```python
from build123d import *

# Parameters (mm, degrees)
SKETCH1_R             = 3.5
BOSS_EXTRUDE1_DEPTH   = 6.35
SKETCH2_R             = 3.25
CUT_EXTRUDE1_DEPTH    = 7.35
LPATTERN1_COUNT       = 5
LPATTERN1_PITCH       = 20
FILLET1_R             = 10
SKETCH3_R             = 3.25
SKETCH3_R_2           = 1
CUT_EXTRUDE2_DEPTH    = 7.35
CHAMFER1_SIZE         = 4
CHAMFER1_SIZE2        = 3.477146951
CHAMFER1_PART_2_SIZE  = 4
CHAMFER1_PART_2_SIZE2 = 3.477146951
CHAMFER1_PART_3_SIZE  = 4
CHAMFER1_PART_3_SIZE2 = 3.477146951
CHAMFER1_PART_4_SIZE  = 4
CHAMFER1_PART_4_SIZE2 = 3.477146951


with BuildPart() as part:
    # Sketch1 → Boss-Extrude1 (new body)
    with BuildSketch(Plane.XY):
        with BuildLine():
            Line((-40, 47.5), (-8.864317001, 107.128594183))
            ThreePointArc((-8.864317001, 107.128594183), (0, 112.5), (8.864317001, 107.128594183))
            Line((8.864317001, 107.128594183), (40, 47.5))
            Line((40, 47.5), (40, -47.5))
            Line((40, -47.5), (-40, -47.5))
            Line((-40, -47.5), (-40, 47.5))
        make_face()
        with Locations((-15, 47.5)):
            Circle(SKETCH1_R, mode=Mode.SUBTRACT)
        with Locations((15, 47.5)):
            Circle(SKETCH1_R, mode=Mode.SUBTRACT)
        with Locations((-15, 27.5)):
            Circle(SKETCH1_R, mode=Mode.SUBTRACT)
        with Locations((15, 27.5)):
            Circle(SKETCH1_R, mode=Mode.SUBTRACT)
    extrude(amount=BOSS_EXTRUDE1_DEPTH)

    # Sketch2 → Cut-Extrude1 (cut, through all)
    with BuildSketch(Plane.XY.offset(6.35)):
        with Locations((30, -37.5)):
            Circle(SKETCH2_R)
        with Locations((-30, -37.5)):
            Circle(SKETCH2_R)
    cut_extrude1 = extrude(amount=-CUT_EXTRUDE1_DEPTH, mode=Mode.SUBTRACT)

    # LPattern1: Cut-Extrude1 ×5
    with Locations(*[(0, i * LPATTERN1_PITCH, 0) for i in range(1, LPATTERN1_COUNT)]):
        add(cut_extrude1, mode=Mode.SUBTRACT)

    # Fillet1
    fillet1_edges = [part.edges().sort_by_distance(p)[0] for p in [
        (40, 47.5, 3.175),
        (40, -47.5, 3.175),
        (-40, -47.5, 3.175),
        (-40, 47.5, 3.175),
    ]]
    fillet(fillet1_edges, radius=FILLET1_R)

    # Sketch3 → Cut-Extrude2 (cut, through all)
    with BuildSketch(Plane.XY.offset(6.35)):
        with Locations((-20, 62.5)):
            Circle(SKETCH3_R)
        with Locations((20, 62.5)):
            Circle(SKETCH3_R)
        with Locations((0, 102.5)):
            Circle(SKETCH3_R_2)
    extrude(amount=-CUT_EXTRUDE2_DEPTH, mode=Mode.SUBTRACT)

    # Chamfer1
    chamfer1_edges = [part.edges().sort_by_distance(p)[0] for p in [
        (-18.5, 47.5, 0),
    ]]
    chamfer1_side = [part.faces().sort_by_distance(p)[0] for p in [
        (-18.5, 47.5, 3.175),
    ]]
    chamfer(chamfer1_edges, length=CHAMFER1_SIZE, length2=CHAMFER1_SIZE2, reference=chamfer1_side[0])

    # Chamfer1 part 2
    chamfer1_part_2_edges = [part.edges().sort_by_distance(p)[0] for p in [
        (11.5, 47.5, 0),
    ]]
    chamfer1_part_2_side = [part.faces().sort_by_distance(p)[0] for p in [
        (11.5, 47.5, 3.175),
    ]]
    chamfer(chamfer1_part_2_edges, length=CHAMFER1_PART_2_SIZE, length2=CHAMFER1_PART_2_SIZE2, reference=chamfer1_part_2_side[0])

    # Chamfer1 part 3
    chamfer1_part_3_edges = [part.edges().sort_by_distance(p)[0] for p in [
        (-18.5, 27.5, 0),
    ]]
    chamfer1_part_3_side = [part.faces().sort_by_distance(p)[0] for p in [
        (-18.5, 27.5, 3.175),
    ]]
    chamfer(chamfer1_part_3_edges, length=CHAMFER1_PART_3_SIZE, length2=CHAMFER1_PART_3_SIZE2, reference=chamfer1_part_3_side[0])

    # Chamfer1 part 4
    chamfer1_part_4_edges = [part.edges().sort_by_distance(p)[0] for p in [
        (11.5, 27.5, 0),
    ]]
    chamfer1_part_4_side = [part.faces().sort_by_distance(p)[0] for p in [
        (11.5, 27.5, 3.175),
    ]]
    chamfer(chamfer1_part_4_edges, length=CHAMFER1_PART_4_SIZE, length2=CHAMFER1_PART_4_SIZE2, reference=chamfer1_part_4_side[0])


solid = part.part
```
Part model, mm, in its own coordinate system. Round coordinates to 2 decimals unless told otherwise and drop trailing zeros. Write each loop counter-clockwise with the first axis right and the second up, starting at its lowest first coordinate (ties: lowest second). Pieces come first, ordered by that corner, then holes.
Item 1: Probe L1, parallel to Y at x = -33, z = 5; L2, parallel to Y at x = -30, z = 3; L3, parallel to X at y = 21, z = 4.5. List the from-to ranges inside material, lowest first.
Results:
L1: y = -47.04 to -38.75, -36.25 to -18.75, -16.25 to 1.25, 3.75 to 21.25, 23.75 to 41.25, 43.75 to 60.91
L2: y = -47.5 to -40.75, -34.25 to -20.75, -14.25 to -0.75, 5.75 to 19.25, 25.75 to 39.25, 45.75 to 66.65
L3: x = -40 to -32.88, -27.12 to 27.12, 32.88 to 40
Item 2: Cut at C-C, the plane z = 1.25. Count the separate pieces of the cut face and the enclosed holes in it, plus the area to 3 significant figures.
Results:
separate pieces: 1
enclosed holes: 17
area: 9,700 mm2
Item 3: Cut at A-A, the plane y = -17.5. Give the cut face in (x, z).
Results:
outline: (-40, 0) - (-33.25, 0) - (-33.25, 6.35) - (-40, 6.35) - close; (-26.75, 0) - (26.75, 0) - (26.75, 6.35) - (-26.75, 6.35) - close; (33.25, 0) - (40, 0) - (40, 6.35) - (33.25, 6.35) - close
Item 4: Cut at D-D, the plane x = 15. Give the cut face in (y, z).
Results:
outline: (-47.5, 0) - (20.52, 0) - (24, 4) - (24, 6.35) - (-47.5, 6.35) - close; (31, 4) - (34.48, 0) - (40.52, 0) - (44, 4) - (44, 6.35) - (31, 6.35) - close; (51, 4) - (54.48, 0) - (95.38, 0) - (95.38, 6.35) - (51, 6.35) - close
Item 5: Drop flat-ended pins along their axis: pin 1 Ø1.5 at (x, z) = (-20.5, 2.5) entering from +Y; pin 2 Ø10.5 at (x, y) = (20, 62.5) entering from -Z. Give the stop position or say it passes through.
Results:
pin 1: stops at y = 86.28
pin 2: stops at z = 0
Item 6: Cut at B-B, the plane x = -28.5. Give the cut face in (y, z), plus the area to 3 significant figures.
Results:
outline: (-47.5, 0) - (-40.38, 0) - (-40.38, 6.35) - (-47.5, 6.35) - close; (-34.62, 0) - (-20.38, 0) - (-20.38, 6.35) - (-34.62, 6.35) - close; (-14.62, 0) - (-0.38, 0) - (-0.38, 6.35) - (-14.62, 6.35) - close; (5.38, 0) - (19.62, 0) - (19.62, 6.35) - (5.38, 6.35) - close; (25.38, 0) - (39.62, 0) - (39.62, 6.35) - (25.38, 6.35) - close; (45.38, 0) - (69.52, 0) - (69.52, 6.35) - (45.38, 6.35) - close
area: 560 mm2
Item 7: Two-plate mould, pull along X, no slides. Class faces 1 (the cylindrical face through (-37.15, -44.49, 3.22)), 2 (the cylindrical face through (39.704, 47.462, 3.219)), 3 (the cylindrical face through (31.5, 39.617, 3.219)), 4 (the cylindrical face through (-0.2, 112.5, 3.1)): +X half, -X half, draft (parallel to the pull), parting line (faces both ways), or undercut.
Results:
face 1: -X half
face 2: +X half
face 3: undercut
face 4: parting line
